Autodesk Inventor part; units mm, degrees
ref_plane "Начальная плоскость" through (0, 0, -10) normal (0, 0, 1) x (1, 0, 0)
ref_plane "Конечная плоскость" through (0, 0, 14) normal (0, 0, 1) x (1, 0, 0)
ref_plane "РабПлоскость4" through (-10, 0, -10) normal (0.7071, 0, -0.7071) x (-0.7071, 0, -0.7071)
ref_plane "Начальная плоскость" through (0, 0, -10) normal (0, 0, 1) x (1, 0, 0)
ref_plane "Конечная плоскость" through (0, 0, 14) normal (0, 0, 1) x (1, 0, 0)
sketch "Эскиз" plane through (0, 0, 0) normal (0, 0, 1) x (1, 0, 0)
  line L0 (-14.4349, 0) -> (14.4349, 0)
  line L1 (0, -14) -> (0, 14)
  line L2 (0, 0) -> (7.5, 7.5) construction
  circle A0 centre (7.5, 7.5) radius 1.65 construction
  line L3 (5.85, 9.15) -> (9.15, 9.15)
  line L4 (9.15, 9.15) -> (9.15, 5.85)
  line L5 (9.15, 5.85) -> (5.85, 5.85)
  line L6 (5.85, 5.85) -> (5.85, 9.15)
  line L7 (3.235, 8.1636) -> (4.72, 9.9636)
  line L8 (4.7971, 10) -> (8.5, 10)
  line L9 (3.3121, 8) -> (4.95, 8)
  line L10 (4.95, 8) -> (4.95, 5.7985)
  line L11 (4.95, 5.7985) -> (2.6515, 3.5)
  line L12 (0, 3.5) -> (2.6515, 3.5)
  circle A1 centre (0, 0) radius 2.5
  line L13 (8.1636, 3.235) -> (9.9636, 4.72)
  line L14 (10, 4.7971) -> (10, 8.5)
  line L15 (8, 3.3121) -> (8, 4.95)
  line L16 (8, 4.95) -> (5.7985, 4.95)
  line L17 (5.7985, 4.95) -> (3.5, 2.6515)
  line L18 (3.5, 0) -> (3.5, 2.6515)
  arc A2 (10, 8.5) -> (8.5, 10) centre (8.5, 8.5) ccw
  line L19 (0, 0) -> (-7.5, 7.5) construction
  circle A3 centre (-7.5, 7.5) radius 1.65 construction
  line L20 (-5.85, 9.15) -> (-9.15, 9.15)
  line L21 (-9.15, 9.15) -> (-9.15, 5.85)
  line L22 (-9.15, 5.85) -> (-5.85, 5.85)
  line L23 (-5.85, 5.85) -> (-5.85, 9.15)
  line L24 (-3.235, 8.1636) -> (-4.72, 9.9636)
  line L25 (-4.7971, 10) -> (-8.5, 10)
  line L26 (-3.3121, 8) -> (-4.95, 8)
  line L27 (-4.95, 8) -> (-4.95, 5.7985)
  line L28 (-4.95, 5.7985) -> (-2.6515, 3.5)
  line L29 (0, 3.5) -> (-2.6515, 3.5)
  line L30 (-3.5, 0) -> (-3.5, 2.6515)
  line L31 (-5.7985, 4.95) -> (-3.5, 2.6515)
  line L32 (-8, 4.95) -> (-5.7985, 4.95)
  line L33 (-8, 3.3121) -> (-8, 4.95)
  line L34 (-8.1636, 3.235) -> (-9.9636, 4.72)
  line L35 (-10, 4.7971) -> (-10, 8.5)
  arc A4 (-8.5, 10) -> (-10, 8.5) centre (-8.5, 8.5) ccw
  line L36 (0, 14) -> (0, -14)
  line L37 (0, 0) -> (7.5, -7.5) construction
  circle A5 centre (7.5, -7.5) radius 1.65 construction
  line L38 (5.85, -9.15) -> (9.15, -9.15)
  line L39 (9.15, -9.15) -> (9.15, -5.85)
  line L40 (9.15, -5.85) -> (5.85, -5.85)
  line L41 (5.85, -5.85) -> (5.85, -9.15)
  line L42 (3.235, -8.1636) -> (4.72, -9.9636)
  line L43 (4.7971, -10) -> (8.5, -10)
  line L44 (3.3121, -8) -> (4.95, -8)
  line L45 (4.95, -8) -> (4.95, -5.7985)
  line L46 (4.95, -5.7985) -> (2.6515, -3.5)
  line L47 (0, -3.5) -> (2.6515, -3.5)
  line L48 (3.5, 0) -> (3.5, -2.6515)
  line L49 (5.7985, -4.95) -> (3.5, -2.6515)
  line L50 (8, -4.95) -> (5.7985, -4.95)
  line L51 (8, -3.3121) -> (8, -4.95)
  line L52 (8.1636, -3.235) -> (9.9636, -4.72)
  line L53 (10, -4.7971) -> (10, -8.5)
  arc A6 (8.5, -10) -> (10, -8.5) centre (8.5, -8.5) ccw
  line L54 (0, 0) -> (-7.5, -7.5) construction
  line L55 (-4.95, -8) -> (-4.95, -5.7985)
  line L56 (-3.3121, -8) -> (-4.95, -8)
  line L57 (-5.7985, -4.95) -> (-3.5, -2.6515)
  line L58 (-4.95, -5.7985) -> (-2.6515, -3.5)
  line L59 (-3.5, 0) -> (-3.5, -2.6515)
  line L60 (0, -3.5) -> (-2.6515, -3.5)
  circle A7 centre (-7.5, -7.5) radius 1.65 construction
  line L61 (-5.85, -5.85) -> (-5.85, -9.15)
  line L62 (-5.85, -9.15) -> (-9.15, -9.15)
  line L63 (-9.15, -9.15) -> (-9.15, -5.85)
  line L64 (-9.15, -5.85) -> (-5.85, -5.85)
  line L65 (-3.235, -8.1636) -> (-4.72, -9.9636)
  line L66 (-8, -4.95) -> (-5.7985, -4.95)
  line L67 (-8, -3.3121) -> (-8, -4.95)
  line L68 (-8.1636, -3.235) -> (-9.9636, -4.72)
  line L69 (-4.7971, -10) -> (-8.5, -10)
  line L70 (-10, -4.7971) -> (-10, -8.5)
  arc A8 (-10, -8.5) -> (-8.5, -10) centre (-8.5, -8.5) ccw
  arc A9 (3.235, 8.1636) -> (3.3121, 8) centre (3.3121, 8.1) ccw
  arc A10 (4.7971, 10) -> (4.72, 9.9636) centre (4.7971, 9.9) ccw
  arc A11 (8, 3.3121) -> (8.1636, 3.235) centre (8.1, 3.3121) ccw
  arc A12 (9.9636, 4.72) -> (10, 4.7971) centre (9.9, 4.7971) ccw
  arc A13 (-3.3121, 8) -> (-3.235, 8.1636) centre (-3.3121, 8.1) ccw
  arc A14 (-4.72, 9.9636) -> (-4.7971, 10) centre (-4.7971, 9.9) ccw
  arc A15 (-8.1636, 3.235) -> (-8, 3.3121) centre (-8.1, 3.3121) ccw
  arc A16 (-10, 4.7971) -> (-9.9636, 4.72) centre (-9.9, 4.7971) ccw
  arc A17 (-8, -3.3121) -> (-8.1636, -3.235) centre (-8.1, -3.3121) ccw
  arc A18 (-9.9636, -4.72) -> (-10, -4.7971) centre (-9.9, -4.7971) ccw
  arc A19 (-3.235, -8.1636) -> (-3.3121, -8) centre (-3.3121, -8.1) ccw
  arc A20 (-4.7971, -10) -> (-4.72, -9.9636) centre (-4.7971, -9.9) ccw
  arc A21 (4.72, -9.9636) -> (4.7971, -10) centre (4.7971, -9.9) ccw
  arc A22 (3.3121, -8) -> (3.235, -8.1636) centre (3.3121, -8.1) ccw
  arc A23 (8.1636, -3.235) -> (8, -3.3121) centre (8.1, -3.3121) ccw
  arc A24 (10, -4.7971) -> (9.9636, -4.72) centre (9.9, -4.7971) ccw
  point P0 (3.1, 8)
  point P1 (4.75, 10)
  point P2 (7.5, 9.15)
  point P3 (8, 3.1)
  point P4 (10, 4.75)
  point P5 (7.5, 5.85)
  point P6 (9.15, 7.5)
  point P7 (-3.1, 8)
  point P8 (-4.75, 10)
  point P9 (-7.5, 9.15)
  point P10 (-8, 3.1)
  point P11 (-10, 4.75)
  point P12 (-7.5, 5.85)
  point P13 (-9.15, 7.5)
  point P14 (3.1, -8)
  point P15 (4.75, -10)
  point P16 (7.5, -9.15)
  point P17 (8, -3.1)
  point P18 (10, -4.75)
  point P19 (7.5, -5.85)
  point P20 (9.15, -7.5)
  point P21 (-3.1, -8)
  point P22 (-7.5, -5.85)
  point P23 (-7.5, -9.15)
  point P24 (-9.15, -7.5)
  point P25 (-4.75, -10)
  point P26 (-8, -3.1)
  point P27 (-10, -4.75)
  dimension "d0" = 45
  dimension "d1" = 3.3
  dimension "d2" = 1.5
  dimension "d3" = 1.2
  dimension "d4" = 5
  dimension "d5" = 6.5
  dimension "d6" = 15
  dimension "d7" = 20
  dimension "d8" = 9.9
  dimension "d9" = 9.5
  dimension "d10" = 6.2
  dimension "d11" = 2
  dimension "d18" = 0.1
  dimension "d19" = 0.1
extrude "Тело" add sketch "Эскиз" along normal up to surface (24 mm away) from surface at -10 contours A1 L1 L12 L11 L10 L9 A9 L7 A10 L8 A2 L14 A12 L13 A11 L15 L16 L17 L18 L0 | L0 L48 L49 L50 L51 A23 L52 A24 L53 A6 L43 A21 L42 A22 L44 L45 L46 L47 L1 A1 | A1 L0 L30 L31 L32 L33 A15 L34 A16 L35 A4 L25 A14 L24 A13 L26 L27 L28 L29 L1 | L1 L60 L58 L55 L56 A19 L65 A20 L69 A8 L70 A18 L68 A17 L67 L66 L57 L59 L0 A1
sketch "Эскиз2" plane through (0, 0, 0) normal (0, 0, 1) x (1, 0, 0)
  line L0 (0, 0) -> (10, 0)
ref_plane "РабПлоскость3" through (0, 0, 0) normal (0, -1, 0) x (1, 0, 0)
sketch "Эскиз3" plane through (0, 0, 0) normal (0, -1, 0) x (1, 0, 0)
  line L0 (-2, -10) -> (12, -10)
  line L1 (-2, 14) -> (12, 14)
  dimension "d25" = 24
ref_plane "РабПлоскость4" through (-10, 0, -10) normal (0.7071, 0, -0.7071) x (-0.7071, 0, -0.7071)
split "Разделение1" plane through (-10, 0, -10) removes the side toward (0.7071, 0, -0.7071)
equation "\"Длина\" = 14"
equation "\"G_OFFSET_END\" = 0"
equation "\"d21\" = Длина + G_OFFSET_END"
equation "\"G_L\" = d25"
properties part number "короткая палка"
Design review of the part built by this model. Coordinates are the model's own, in mm. A direction names the side the tool comes from. Coordinates: 2 decimals unless noted, no trailing zeros. Order: outer loops, then holes, each group sorted by start corner. A loop starts at its lowest first (then second) coordinate and runs counter-clockwise, first axis right, second up.
Item 1: For faces 1 (the flat face through (-10, -7, 2)), 2 (the flat face through (-4, -8, 4)), 3 (the flat face through (-3.5, 0, 5)), 4 (the cylindrical face through (-9.55, -9.57, 1.83)), 5 (the flat face through (3.967, -9.051, 8.542)), list the 3-axis set-ups (+Z, -Z, +X, -X, +Y, -Y) from which the entire face can be reached by the end or side of a thin tool; tool diameter is ignored.
Item 2: Take a section at B-B, the plane x = 0. Write out the cut boundary in (y, z).
Item 3: For line 1 (Y direction, x = -7, z = 10); line 2 (X direction, y = 0, z = 4.5), list the stretches that pass through material, from the lowest coordinate up.
Item 4: Take a section at C-C, the plane z = 11.5. Count the separate pieces of the cut face and the enclosed holes in it, then the cut area to 3 significant figures.
Item 5: Take a section at A-A, the plane y = -1.5. Write out the cut boundary in (x, z).
Item 6: For pin 1 Ø2.5 at (y, z) = (8, 1.5) entering from +X; pin 2 Ø0.5 at (y, z) = (-4, 10) entering from -X; pin 3 Ø1.5 at (x, z) = (-0.5, -1) entering from -Y, all flat-tipped, find the tip position at first contact; note any pin that passes through.
Item 7: The part is to be moulded in two halves that separate along X. For faces 6 (the flat face through (10, 7, 12)), 7 (the flat face through (-4, 8, 4)), 8 (the flat face through (-9.051, -3.967, 1.85)), say which applies: pulls with the +X half, pulls with the -X half, needs draft (parallel to the pull), parting line crosses it, or undercut.
The answers:
1. face 1: +Z, -Z, -X, +Y, -Y
1. face 2: +Z, -Z
1. face 3: +Z, -Z, -X
1. face 4: +Z, -Z, -X, -Y
1. face 5: +Z, -Z, -Y
2. outline: (-3.5, 0) - (-2.5, 0) - (-2.5, 14) - (-3.5, 14) - close; (2.5, 0) - (3.5, 0) - (3.5, 14) - (2.5, 14) - close
3. line 1: y = -10 to -9.15, -5.85 to -4.95, 4.95 to 5.85, 9.15 to 10
3. line 2: x = -3.5 to -2.5, 2.5 to 3.5
4. separate pieces: 1
4. enclosed holes: 5
4. area: 115 mm2
5. outline: (-3.5, -3.5) - (-2, -2) - (-2, 14) - (-3.5, 14) - close; (2, 2) - (3.5, 3.5) - (3.5, 14) - (2, 14) - close
6. pin 1: stops at x = -3.21
6. pin 2: stops at x = -9.39
6. pin 3: stops at y = -3.5
7. face 6: pulls with the +X half
7. face 7: undercut
7. face 8: pulls with the -X half
